Work out the finished part from the listing and answer in its coordinate system (mm). A direction names the side the tool comes from. Coordinates: 2 decimals unless noted, no trailing zeros. Order: outer loops, then holes, each group sorted by start corner. A loop starts at its lowest first (then second) coordinate and runs counter-clockwise, first axis right, second up. Notation, with made-up numbers: (-38, 79.5) - (-30, 79.5) arc R13 cw to (-30, 83.5) - close; hole circle Ø1 at (-26, 7.5). An arc over 180 degrees is marked (long way). Answer as a JSON object with one key per item and string values. Group by question number.
1) A tool of negligible diameter and unlimited length cuts with its end or side. For faces 1 (the face through (163, 0, -119)), 2 (the face through (218.39, 2.47, -128.68)), from which of +Z, -Z, +X, -X, +Y, -Y can it reach the whole face along a straight path? Write none if from no direction.
2) The mould has two halves that part along Z. Classify faces 3 (the face through (163, 5, -119)), 4 (the face through (219.107, 2.465, -63.733)): released by +Z, released by -Z, zero draft, split by the parting line, or undercut.
3) Section A-A (x = 96) is taken. Give the vertices of the cut face in (y, z), plus the area to 3 significant figures.
4) Section B-B (y = 2.3) is taken. Count the separate pieces of the cut face and the enclosed holes in it, plus the area to 3 significant figures.
5) Find the intervals of material crossed by line 1 along X through (y, z) = (2.3, -46.5); line 2 along Z through (x, y) = (10, 2.75); line 3 along X through (y, z) = (1.3, -96), in increasing order.
6) Each of these flat-tipped pins is pushed along its axis until it touches: P1, Ø2.5, axis at x = 47.96, z = -78.59, coming from the -Y side; P2, Ø2.5, axis at y = 3.5, z = -119.5, coming from the -X side; P3, Ø2, axis at y = 1, z = -36, coming from the +X side. Where does it stop, or does it pass through?
from build123d import *

# Parameters (mm, degrees)
SKETCH1_W                = 330
SKETCH1_H                = 192
BOSS_EXTRUDE1_DEPTH      = 5
CUT_EXTRUDE1_DEPTH       = 382.823257542
CUT_EXTRUDE1_DEPTH_BACK  = 382.823257542
SKETCH2_R                = 1.5
SKETCH3_R                = 41.5
CUT_EXTRUDE2_DEPTH       = 382.823257542
M5_CLEARANCE_HOLE1_D     = 5.3
M5_CLEARANCE_HOLE1_DEPTH = 11.94
M5_CLEARANCE_HOLE1_TIP   = 1.59228064
TAP_DRILL_FOR_M4_TAP1_D  = 3.3
CUT_EXTRUDE3_DEPTH       = 382.823257542
CUT_EXTRUDE3_DEPTH_BACK  = 382.823257542
SKETCH19_W               = 28
SKETCH19_H               = 120
SKETCH21_W               = 55
SKETCH21_H               = 89
CUT_EXTRUDE4_DEPTH       = 382.823257542
FILLET1_R                = 4
TAP_DRILL_FOR_M3_TAP1_D  = 2.5
TAP_DRILL_FOR_M3_TAP2_D  = 2.5
CUT_EXTRUDE5_DEPTH       = 382.823257542
FILLET2_R                = 4
SKETCH33_W               = 98
SKETCH33_H               = 30
CUT_EXTRUDE6_DEPTH       = 382.82325768
FILLET3_R                = 5


with BuildPart() as part:
    # Sketch1 → Boss-Extrude1 (new body)
    with BuildSketch(Plane(origin=(0, 0, 0), x_dir=(1, 0, 0), z_dir=(0, 1, 0))):
        with Locations((165, 96)):
            Rectangle(SKETCH1_W, SKETCH1_H)
    extrude(amount=BOSS_EXTRUDE1_DEPTH)

    # Sketch2 → Cut-Extrude1 (cut, two sides: drawn at the far end of the back side and taken through both)
    with BuildSketch(Plane(origin=(0, 5, 0), x_dir=(1, 0, 0), z_dir=(0, 1, 0)).offset(-CUT_EXTRUDE1_DEPTH_BACK)):
        with Locations(Location((132.036518729, 113.412096173, 0), (0, 0, 270))):
            Circle(SKETCH2_R)
        with Locations(Location((132.036518729, 78.587903827, 0), (0, 0, 270))):
            Circle(SKETCH2_R)
        with Locations(Location((107.412096173, 53.963481271, 0), (0, 0, 270))):
            Circle(SKETCH2_R)
        with Locations(Location((72.587903827, 53.963481271, 0), (0, 0, 270))):
            Circle(SKETCH2_R)
        with Locations(Location((47.963481271, 78.587903827, 0), (0, 0, 270))):
            Circle(SKETCH2_R)
        with Locations(Location((47.963481271, 113.412096173, 0), (0, 0, 270))):
            Circle(SKETCH2_R)
        with Locations(Location((72.587903827, 138.036518729, 0), (0, 0, 270))):
            Circle(SKETCH2_R)
        with Locations(Location((107.412096173, 138.036518729, 0), (0, 0, 270))):
            Circle(SKETCH2_R)
    extrude(amount=CUT_EXTRUDE1_DEPTH + CUT_EXTRUDE1_DEPTH_BACK, mode=Mode.SUBTRACT)

    # Sketch3 → Cut-Extrude2 (cut, through all)
    with BuildSketch(Plane(origin=(0, 5, 0), x_dir=(1, 0, 0), z_dir=(0, 1, 0))):
        with Locations(Location((90, 96, 0), (0, 0, 270))):
            Circle(SKETCH3_R)
    extrude(amount=-CUT_EXTRUDE2_DEPTH, mode=Mode.SUBTRACT)

    # M5 Clearance Hole1
    with Locations(Plane(origin=(0, 5, 0), x_dir=(1, 0, 0), z_dir=(0, 1, 0))):
        with Locations((10, 172), (10, 10), (320, 10), (320, 172)):
            Hole(M5_CLEARANCE_HOLE1_D / 2, depth=M5_CLEARANCE_HOLE1_DEPTH)
            with Locations((0, 0, -(M5_CLEARANCE_HOLE1_DEPTH + M5_CLEARANCE_HOLE1_TIP / 2))):  # 118° drill point
                Cone(0, M5_CLEARANCE_HOLE1_D / 2, M5_CLEARANCE_HOLE1_TIP, mode=Mode.SUBTRACT)

    # Tap Drill for M4 Tap1 (through all)
    with Locations(Plane(origin=(0, 5, 0), x_dir=(1, 0, 0), z_dir=(0, 1, 0))):
        with Locations((137.5, 96), (90, 48.5), (42.5, 96), (90, 143.5)):
            Hole(TAP_DRILL_FOR_M4_TAP1_D / 2)

    # Sketch19 → Cut-Extrude3 (cut, two sides: drawn at the far end of the back side and taken through both)
    with BuildSketch(Plane(origin=(0, 5, 0), x_dir=(1, 0, 0), z_dir=(0, 1, 0)).offset(-CUT_EXTRUDE3_DEPTH_BACK)):
        with Locations((14, 96)):
            Rectangle(SKETCH19_W, SKETCH19_H)
        with Locations((316, 96)):
            Rectangle(SKETCH19_W, SKETCH19_H)
    extrude(amount=CUT_EXTRUDE3_DEPTH + CUT_EXTRUDE3_DEPTH_BACK, mode=Mode.SUBTRACT)

    # Sketch21 → Cut-Extrude4 (cut, through all)
    with BuildSketch(Plane.XZ):
        with Locations((274.5, -96)):
            Rectangle(SKETCH21_W, SKETCH21_H)
    extrude(amount=-CUT_EXTRUDE4_DEPTH, mode=Mode.SUBTRACT)

    # Fillet1
    fillet1_edges = [part.edges().sort_by_distance(p)[0] for p in [
        (0, 2.5, -36),
        (0, 2.5, -156),
        (28, 2.5, -156),
        (28, 2.5, -36),
        (330, 2.5, -156),
        (330, 2.5, -36),
        (302, 2.5, -36),
        (302, 2.5, -156),
        (302, 2.5, -51.5),
        (302, 2.5, -140.5),
        (247, 2.5, -140.5),
        (247, 2.5, -51.5),
    ]]
    fillet(fillet1_edges, radius=FILLET1_R)

    # Tap Drill for M3 Tap1 (through all)
    with Locations(Plane(origin=(0, 0, 0), x_dir=(-1, 0, 0), z_dir=(0, -1, 0))):
        with Locations((-182.5, 126.310889132), (-182.5, 65.689110868), (-235, 96)):
            Hole(TAP_DRILL_FOR_M3_TAP1_D / 2)

    # Tap Drill for M3 Tap2 (through all)
    with Locations(Plane(origin=(0, 0, 0), x_dir=(-1, 0, 0), z_dir=(0, -1, 0))):
        with Locations((-154, 46.5), (-136, 46.5)):
            Hole(TAP_DRILL_FOR_M3_TAP2_D / 2)

    # Sketch32 → Cut-Extrude5 (cut, through all)
    with BuildSketch(Plane.XZ):
        with BuildLine():
            ThreePointArc((237.232142857, -100.474096363), (230, -96), (237.232142857, -91.525903637))
            ThreePointArc((237.232142857, -91.525903637), (218.75, -63.524047358), (185.258609681, -61.518970267))
            ThreePointArc((185.258609681, -61.518970267), (186.904148522, -63.321944672), (187.5, -65.689110868))
            ThreePointArc((187.5, -65.689110868), (182.6520482, -70.686798467), (177.509247462, -65.99306663))
            ThreePointArc((177.509247462, -65.99306663), (162.5, -96), (177.509247462, -126.00693337))
            ThreePointArc((177.509247462, -126.00693337), (182.6520482, -121.313201533), (187.5, -126.310889132))
            ThreePointArc((187.5, -126.310889132), (186.904148522, -128.678055328), (185.258609681, -130.481029733))
            ThreePointArc((185.258609681, -130.481029733), (218.75, -128.475952642), (237.232142857, -100.474096363))
        make_face()
    extrude(amount=-CUT_EXTRUDE5_DEPTH, mode=Mode.SUBTRACT)

    # Fillet2
    fillet2_edges = [part.edges().sort_by_distance(p)[0] for p in [
        (237.232142857, 2.5, -91.525903637),
        (237.232142857, 2.5, -100.474096363),
        (185.258609681, 2.5, -130.481029733),
        (177.509247462, 2.5, -126.00693337),
        (177.509247462, 2.5, -65.99306663),
        (185.258609681, 2.5, -61.518970267),
    ]]
    fillet(fillet2_edges, radius=FILLET2_R)

    # Sketch33 → Cut-Extrude6 (cut, through all)
    with BuildSketch(Plane.XZ):
        with Locations((105, -15)):
            Rectangle(SKETCH33_W, SKETCH33_H)
        with Locations((105, -177)):
            Rectangle(SKETCH33_W, SKETCH33_H)
    extrude(amount=-CUT_EXTRUDE6_DEPTH, mode=Mode.SUBTRACT)

    # Fillet3
    fillet3_edges = [part.edges().sort_by_distance(p)[0] for p in [
        (56, 2.5, -30),
        (56, 2.5, 0),
        (154, 2.5, 0),
        (154, 2.5, -30),
        (56, 2.5, -192),
        (56, 2.5, -162),
        (154, 2.5, -162),
        (154, 2.5, -192),
        (0, 2.5, -192),
        (330, 2.5, -192),
        (330, 2.5, 0),
        (0, 2.5, 0),
    ]]
    fillet(fillet3_edges, radius=FILLET3_R)


solid = part.part
Report:
{
 "1": {"face 1": "+Z, -Z, +X, -X, -Y", "face 2": "+Y, -Y"},
 "2": {"face 3": "zero draft", "face 4": "undercut"},
 "3": {"outline": "(0, -162) - (5, -162) - (5, -137.06) - (0, -137.06) - close; (0, -54.94) - (5, -54.94) - (5, -30) - (0, -30) - close", "area": "249 mm²"},
 "4": {"separate pieces": "1", "enclosed holes": "23", "area": "36,000 mm²"},
 "5": {"line 1": "x = 28 to 134.75, 137.25 to 152.75, 155.25 to 302", "line 2": "z = -192 to -174.65, -169.35 to -156, -36 to -12.65, -7.35 to 0", "line 3": "x = 28 to 40.85, 44.15 to 48.5, 131.5 to 135.85, 139.15 to 162.5, 230 to 233.75, 236.25 to 247"},
 "6": {"P1": "passes through", "P2": "stops at x = 28", "P3": "stops at x = 328.65"}
}
